Input: part model. Units: mm. Frame: model coordinates. A direction names the side the tool comes from. Round coordinates to 2 decimals unless told otherwise and drop trailing zeros. Order: outer loops, then holes, each group sorted by start corner. A loop starts at its lowest first (then second) coordinate and runs counter-clockwise, first axis right, second up. Notation, with made-up numbers: M 46.5,-26 L 81.5,-26 A20 cw 81.5,-17 Z; hole C 56.25,55.5 d5. An arc over 180 degrees is marked long. One line per question, with ' | ' between items.
```python
from build123d import *

# Parameters (mm, degrees)
SKETCH1_R                            = 2.0193
BOSS_EXTRUDE1_DEPTH                  = 14.2875
F_10_32_TAPPED_HOLE1_D               = 4.0386
F_10_32_TAPPED_HOLE1_DEPTH           = 11.938
F_10_32_TAPPED_HOLE1_TIP             = 1.213317848
F_10_32_TAPPED_HOLE1_ON_FACE_2_D     = 4.0386
F_10_32_TAPPED_HOLE1_ON_FACE_2_DEPTH = 11.938
F_10_32_TAPPED_HOLE1_ON_FACE_2_TIP   = 1.213317848
SKETCH4_R                            = 8.89
SKETCH4_R_2                          = 6.35
CUT_EXTRUDE_THIN1_DEPTH              = 7.9375


with BuildPart() as part:
    # Sketch1 → Boss-Extrude1 (new, symmetric)
    with BuildSketch(Plane.XY):
        with BuildLine():
            ThreePointArc((6.874999966, 0), (6.860422465, 0.447468582), (6.816751782, 0.893039571))
            Line((6.816751782, 0.893039571), (4.181770846, 5.456960429))
            ThreePointArc((4.181770846, 5.456960429), (3.437499983, 5.953924622), (2.634980936, 6.35))
            Line((2.634980936, 6.35), (-2.634980936, 6.35))
            ThreePointArc((-2.634980936, 6.35), (-3.437499983, 5.953924622), (-4.181770846, 5.456960429))
            Line((-4.181770846, 5.456960429), (-6.816751782, 0.893039571))
            ThreePointArc((-6.816751782, 0.893039571), (-6.874999966, 0), (-6.816751782, -0.893039571))
            Line((-6.816751782, -0.893039571), (-4.181770846, -5.456960429))
            ThreePointArc((-4.181770846, -5.456960429), (-3.437499983, -5.953924622), (-2.634980936, -6.35))
            Line((-2.634980936, -6.35), (2.634980936, -6.35))
            ThreePointArc((2.634980936, -6.35), (3.437499983, -5.953924622), (4.181770846, -5.456960429))
            Line((4.181770846, -5.456960429), (6.816751782, -0.893039571))
            ThreePointArc((6.816751782, -0.893039571), (6.860422465, -0.447468582), (6.874999966, 0))
        make_face()
        Circle(SKETCH1_R, mode=Mode.SUBTRACT)
    extrude(amount=BOSS_EXTRUDE1_DEPTH, both=True)

    # #10-32 Tapped Hole1
    with Locations(Plane.XY.offset(14.2875)):
        with Locations((0, 0)):
            Hole(F_10_32_TAPPED_HOLE1_D / 2, depth=F_10_32_TAPPED_HOLE1_DEPTH)
            with Locations((0, 0, -(F_10_32_TAPPED_HOLE1_DEPTH + F_10_32_TAPPED_HOLE1_TIP / 2))):  # 118° drill point
                Cone(0, F_10_32_TAPPED_HOLE1_D / 2, F_10_32_TAPPED_HOLE1_TIP, mode=Mode.SUBTRACT)

    # #10-32 Tapped Hole1 on face 2
    with Locations(Plane.XY.offset(-14.2875)):
        with Locations((0, 0)):
            Hole(F_10_32_TAPPED_HOLE1_ON_FACE_2_D / 2, depth=F_10_32_TAPPED_HOLE1_ON_FACE_2_DEPTH)
            with Locations((0, 0, -(F_10_32_TAPPED_HOLE1_ON_FACE_2_DEPTH + F_10_32_TAPPED_HOLE1_ON_FACE_2_TIP / 2))):  # 118° drill point
                Cone(0, F_10_32_TAPPED_HOLE1_ON_FACE_2_D / 2, F_10_32_TAPPED_HOLE1_ON_FACE_2_TIP, mode=Mode.SUBTRACT)

    # Sketch4 → Cut-Extrude-Thin1 (cut)
    with BuildSketch(Plane.XY.offset(14.2875)):
        Circle(SKETCH4_R)
        Circle(SKETCH4_R_2, mode=Mode.SUBTRACT)
    cut_extrude_thin1 = extrude(amount=-CUT_EXTRUDE_THIN1_DEPTH, mode=Mode.SUBTRACT)

    # Mirror1: Cut-Extrude-Thin1 across plane
    add(cut_extrude_thin1.mirror(Plane.XY), mode=Mode.SUBTRACT)


solid = part.part
```
Item 1: Line query: line 1 along Y through (x, z) = (0, 8.25); line 2 along Y through (x, z) = (1, -8); line 3 along Y through (x, z) = (5.5, -3). Output: solid intervals per line, ascending. Write a range as from..to.
Report:
line 1: -6.35..-2.02, 2.02..6.35 | line 2: -6.27..-1.75, 1.75..6.27 | line 3: -3.17..3.17
Item 2: Section query C-C, the plane y = 4. Return loops of the section in (x, z).
Report:
outline: M -5.02,-6.35 L -4.93,-6.35 L -4.93,-14.29 L 4.93,-14.29 L 4.93,-6.35 L 5.02,-6.35 L 5.02,6.35 L 4.93,6.35 L 4.93,14.29 L -4.93,14.29 L -4.93,6.35 L -5.02,6.35 Z
Item 3: Section query D-D, the plane z = -9.5. Return loops of the section in (x, y).
Report:
outline: C 0,0 d12.7; hole C 0,0 d4.04
Item 4: Section query B-B, the plane x = -4.5. Return loops of the section in (y, z).
Report:
outline: M -4.91,-6.35 L -4.48,-6.35 L -4.48,-14.29 L 4.48,-14.29 L 4.48,-6.35 L 4.91,-6.35 L 4.91,6.35 L 4.48,6.35 L 4.48,14.29 L -4.48,14.29 L -4.48,6.35 L -4.91,6.35 Z
Item 5: Section query A-A, the plane z = 4.5. Return loops of the section in (x, y) (3 decimals), plus the area to 3 significant figures.
Report:
outline: M -6.817,-0.893 L -4.182,-5.457 A6.875 ccw -2.635,-6.35 L 2.635,-6.35 A6.875 ccw 4.182,-5.457 L 6.817,-0.893 A6.875 ccw 6.817,0.893 L 4.182,5.457 A6.875 ccw 2.635,6.35 L -2.635,6.35 A6.875 ccw -4.182,5.457 L -6.817,0.893 A6.875 ccw Z; hole C 0,0 d4.039 | area: 125 mm²
Item 6: Access query for faces 1 (the flat face through (3, 6, -6.35)), 2 (the flat face through (6.5, 0, -6.35)), 3 (the flat face through (3, -6, -6.35)), 4 (the cylindrical face through (-1.38, -6.2, 10.37)). Directions: +Z, -Z, +X, -X, +Y, -Y. A direction counts if a zero-diameter tool reaches every point of the face in a straight line with its end or side. Return the directions, or none.
Report:
face 1: -Z, +X, +Y | face 2: -Z, +X | face 3: -Z, +X, -Y | face 4: +Z
Item 7: First-contact query: pin 1 (1.5 mm diameter, centred on y = 3, z = -7, fed in from -X); pin 2 (6 mm diameter, centred on y = 2.5, z = -9.5, fed in from -X); pin 3 (2 mm diameter, centred on x = -0.5, y = 0.5, fed in from +Z). Flat tips, straight axial feed; report the tip coordinate or a pass-through.
Report:
pin 1: x = -5.94 | pin 2: x = -6.35 | pin 3: through
